from build123d import *

# Parameters (mm, degrees)
SKETCH1_W                    = 44.45
SKETCH1_H                    = 12.7
BOSS_EXTRUDE1_DEPTH          = 457.2
SKETCH2_W                    = 38.1
SKETCH2_H                    = 9.525
CUT_EXTRUDE1_DEPTH           = 457.2
F_10_0_1935_DIAMETER_HOLE3_D = 4.9149


with BuildPart() as part:
    # Sketch1 → Boss-Extrude1 (new body)
    with BuildSketch(Plane(origin=(0, 0, 0), x_dir=(0, 0, -1), z_dir=(1, 0, 0))):
        with Locations((22.225, 6.35)):
            Rectangle(SKETCH1_W, SKETCH1_H)
    extrude(amount=BOSS_EXTRUDE1_DEPTH)

    # Sketch2 → Cut-Extrude1 (cut)
    with BuildSketch(Plane.ZY):
        with Locations((-22.225, 7.9375)):
            Rectangle(SKETCH2_W, SKETCH2_H)
    extrude(amount=-CUT_EXTRUDE1_DEPTH, mode=Mode.SUBTRACT)

    # #10 (0.1935) Diameter Hole3 (through all)
    with Locations(Plane(origin=(450.832652449, 0, -31.016622241), x_dir=(0, 0, -1), z_dir=(0, -1, 0))):
        with Locations((0, 0), (-25.407873942, -0.017970114), (0.032060561, -444.542685672), (-25.413373891, -444.602634996)):
            Hole(F_10_0_1935_DIAMETER_HOLE3_D / 2)


solid = part.part
The model under review builds one solid part; all positions refer to its coordinate system, in mm. A direction names the side the tool comes from. Round coordinates to 2 decimals unless told otherwise and drop trailing zeros. Order: outer loops, then holes, each group sorted by start corner. A loop starts at its lowest first (then second) coordinate and runs counter-clockwise, first axis right, second up. Notation, with made-up numbers: (40, 55) -> (77, 55) arc R15 ccw to (77, 82) -> close; hole circle Ø11 at (-12, 4.25). An arc over 180 degrees is marked (long way). Write item = value, one per line. Start each with the question number.
Item 1: For faces 1 (the face through (457.2, 2, -22)), 2 (the face through (225, 3.175, -22)), list the 3-axis set-ups (+Z, -Z, +X, -X, +Y, -Y) from which the entire face can be reached by the end or side of a thin tool; tool diameter is ignored.
Item 2: Consider section C-C on z = -12. Write out the cut boundary in (x, y) (3 decimals), plus the area to 3 significant figures.
Item 3: Consider section A-A on y = 7. Write out the cut boundary in (x, z) (3 decimals), plus the area to 3 significant figures.
Item 4: Clearance check with flat-ended pins moving along their axes: pin 1 Ø11.5 at (x, z) = (273.5, -22.5) entering from +Y (3 decimals); pin 2 Ø8 at (x, z) = (6.23, -5.6) entering from -Y; pin 3 Ø4.5 at (x, z) = (6.29, -31.05) entering from -Y. State where each tip first meets the part, or that it passes through.
Item 5: Mouldability with a two-part tool opening along Z and no side actions: class faces 3 (the face through (225, 6, -44.45)), 4 (the face through (225, 8, -3.175)), 5 (the face through (225, 8, -41.275)), 6 (the face through (0, 2, -22)) as released by +Z, released by -Z, zero draft, split by the parting line, or undercut.
Item 6: For line 1 along X through (y, z) = (1.5, -5); line 2 along Z through (x, y) = (177.5, 10) (3 decimals); line 3 along Y through (x, z) = (391, -24) (3 decimals), list the stretches that pass through material, from the lowest coordinate up.
Item 7: Consider section B-B on x = 365. Write out the cut boundary in (y, z) (3 decimals), plus the area to 3 significant figures.
Conclusion:
q1.face_1 = +Z, -Z, +X, +Y, -Y
q1.face_2 = +X, -X, +Y
q2.outline = (0, 0) -> (457.2, 0) -> (457.2, 3.175) -> (0, 3.175) -> close
q2.area = 1,450 mm2
q3.outline = (0, -44.45) -> (457.2, -44.45) -> (457.2, -41.275) -> (0, -41.275) -> close; (0, -3.175) -> (5.852, -3.175) arc R2.457 cw to (6.608, -3.175) -> (450.474, -3.175) arc R2.457 cw to (451.155, -3.175) -> (457.2, -3.175) -> (457.2, 0) -> (0, 0) -> close
q3.area = 2,900 mm2
q4.pin_1 = 3.175
q4.pin_2 = 0
q4.pin_3 = through
q5.face_3 = released by -Z
q5.face_4 = undercut
q5.face_5 = undercut
q5.face_6 = zero draft
q6.line_1 = 0 to 3.85, 8.61 to 448.43, 453.2 to 457.2
q6.line_2 = -44.45 to -41.275, -3.175 to 0
q6.line_3 = 0 to 3.175
q7.outline = (0, -44.45) -> (12.7, -44.45) -> (12.7, -41.275) -> (3.175, -41.275) -> (3.175, -3.175) -> (12.7, -3.175) -> (12.7, 0) -> (0, 0) -> close
q7.area = 202 mm2
